Work out the finished part from the listing and answer in its coordinate system (mm). Face numbers are marked on the shaded views. A direction names the side the tool comes from. Give positions to 0.01 mm unless a question says otherwise; leave off trailing zeros. Order: outer loops, then holes, each group sorted by start corner. A loop starts at its lowest first (then second) coordinate and runs counter-clockwise, first axis right, second up.
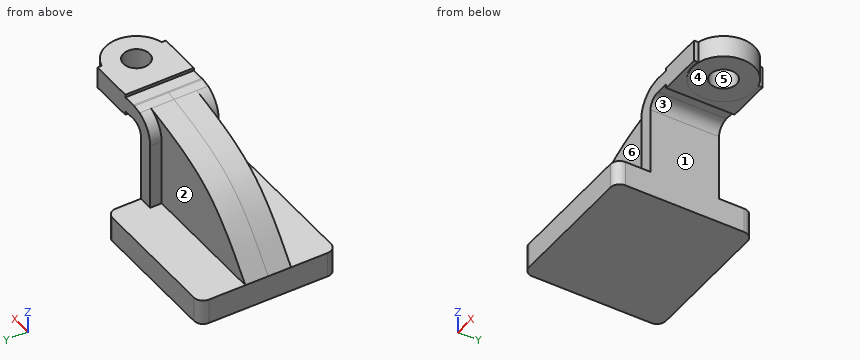
```python
from build123d import *

# Parameters (mm, degrees)
F1_DEPTH = 38.1
F2_DEPTH = 19.05
F3_DEPTH = 12.7
F5_DEPTH = 12.192
F6_R     = 5.08
F7_R     = 7.266587331
F8_DEPTH = 67.1105764264


with BuildPart() as f1:
    # F0 (on Front) → F1 (new body, symmetric)
    with BuildSketch(Plane.XZ):
        Polygon((-40.8368967474, -6.9965338334), (40.8368967474, -6.9965338334), (40.8368967474, 6.9965338334), (32.7088981867, 6.9965338334), (-40.8368967474, 6.9965338334), align=None)
    extrude(amount=F1_DEPTH, both=True)

    # F0 (on Front) → F2 (join, symmetric)
    with BuildSketch(Plane.XZ):
        with BuildLine():
            Line((32.7088981867, 6.9965338334), (40.8368967474, 6.9965338334))
            Line((40.8368967474, 6.9965338334), (40.8368967474, 44.1209748387))
            ThreePointArc((40.8368967474, 44.1209748387), (42.7787364938, 48.6655280984), (47.405064106, 50.403572619))
            Line((47.405064106, 50.403572619), (54.5443966985, 50.403572619))
            Line((54.5443966985, 50.403572619), (54.5443966985, 58.5315711796))
            Line((54.5443966985, 58.5315711796), (47.5487387444, 58.5315711796))
            ThreePointArc((47.5487387444, 58.5315711796), (47.1257024985, 58.5377791506), (46.7026662526, 58.5315711796))
            add(Edge.make_bspline(
                [(42.0115930359, 57.6002229992), (43.5737310544, 57.9125891747), (45.1381986535, 58.2220801772), (46.7026662526, 58.5315711796)],
                knots=[0.9578817781, 0.9578817781, 0.9578817781, 0.9578817781, 1, 1, 1, 1], degree=3))
            ThreePointArc((42.0115930359, 57.6002229992), (35.2603461634, 52.3098432347), (32.7088981867, 44.1209748387))
            Line((32.7088981867, 44.1209748387), (32.7088981867, 6.9965338334))
        make_face()
        Polygon((54.5443966985, 58.5315711796), (54.5443966985, 50.403572619), (54.5443966985, 48.1189936399), (79.1036263108, 48.1189936399), (79.1036263108, 60.113042593), (54.5443966985, 60.113042593), align=None)
    extrude(amount=F2_DEPTH, both=True)

    # F0 (on Front) → F3 (join, symmetric)
    with BuildSketch(Plane.XZ):
        with BuildLine():
            add(Edge.make_bspline(
                [(-40.8368967474, 6.9965338334), (-30.668528225, 20.158177618), (-10.5181051355, 46.2403057616), (24.4122257068, 54.0810415955), (42.0115930359, 57.6002229992)],
                knots=[0, 0, 0, 0, 0.4833692512, 0.9578817781, 0.9578817781, 0.9578817781, 0.9578817781], degree=3))
            Line((-40.8368967474, 6.9965338334), (32.7088981867, 6.9965338334))
            Line((32.7088981867, 6.9965338334), (32.7088981867, 44.1209748387))
            ThreePointArc((32.7088981867, 44.1209748387), (35.2603461634, 52.3098432347), (42.0115930359, 57.6002229992))
        make_face()
    extrude(amount=F3_DEPTH, both=True)

    # F4 (on face) → F5 (join)
    with BuildSketch(Plane.XY.offset(60.113042593)):
        with BuildLine():
            Line((79.1036263108, -16.6910297118), (79.1036263108, 16.6910297118))
            ThreePointArc((79.1036263108, 16.6910297118), (57.6104526514, 0), (79.1036263108, -16.6910297118))
        make_face()
        with BuildLine():
            ThreePointArc((79.1036263108, -16.6910297118), (88.4444418904, -10.5664449916), (92.0654381519, 0))
            ThreePointArc((92.0654381519, 0), (88.4444418904, 10.5664449916), (79.1036263108, 16.6910297118))
            Line((79.1036263108, 16.6910297118), (79.1036263108, -16.6910297118))
        make_face()
    extrude(amount=-F5_DEPTH)

    # F6
    f6_edges = [f1.edges().sort_by_distance(p)[0] for p in [
        (-40.836897, -38.1, 0),
        (40.836897, -38.1, 0),
        (40.836897, 38.1, 0),
        (-40.836897, 38.1, 0),
    ]]
    fillet(f6_edges, radius=F6_R)

    # F7 (on face) → F8 (cut, through all)
    with BuildSketch(Plane.XY.offset(60.113042593)):
        with Locations((74.8379454017, 0)):
            Circle(F7_R)
    extrude(amount=-F8_DEPTH, mode=Mode.SUBTRACT)


solid = f1.part
```
1. The part is cut by section C-C (y = 24). Write down the section's boundary in (x, z), then the cut area to 3 significant figures.
Findings below:
outline: (-40.84, -7) - (40.84, -7) - (40.84, 7) - (-40.84, 7) - close
area: 1,140 mm2
2. Straight lines are drawn through the part: probe 1 along Z at (x, y) = (-2.5, 20); probe 2 along Y at (x, z) = (40, 39.5); probe 3 along Y at (x, z) = (-14, 34.5). For each, find the intervals that lie inside material, in ascending order.
Findings below:
probe 1: z = -7 to 7
probe 2: y = -19.05 to 19.05
probe 3: y = -12.7 to 12.7
3. Given P1, Ø1.9, axis at y = -15.5, z = 28, coming from the -X side; P2, Ø10, axis at x = 43.5, y = 7.5, coming from the +Z side; P3, Ø17, axis at x = 67, y = 3.5, coming from the -Z side; P4, Ø2, axis at x = 58.5, y = -20, coming from the +Z side, each flat-ended and moving along its own axis, determine where each tip first touches the part or whether it passes through.
Findings below:
P1: stops at x = 32.71
P2: stops at z = 58.54
P3: stops at z = 47.92
P4: stops at z = 60.11
4. Which of the six approach directions +Z, -Z, +X, -X, +Y, -Y give full straight-line access (tool end or side, diameter ignored) to the marked faces 1, 2 and 3?
Findings below:
face 1: -Z, +X, +Y, -Y
face 2: +Z, -X, +Y
face 3: -Z, +Y, -Y
5. The part is cut by section A-A (x = 74). Write down the section's boundary in (y, z), then the cut area to 3 significant figures.
Findings below:
outline: (-19.05, 48.12) - (-17.21, 48.12) - (-17.21, 47.92) - (-7.22, 47.92) - (-7.22, 60.11) - (-19.05, 60.11) - close; (7.22, 47.92) - (17.21, 47.92) - (17.21, 48.12) - (19.05, 48.12) - (19.05, 60.11) - (7.22, 60.11) - close
area: 288 mm2
6. The mould has two halves that part along Y. Classify the marked faces 4, 5 and 6: pulls with the +Y half, pulls with the -Y half, needs draft (parallel to the pull), parting line crosses it, or undercut.
Findings below:
face 4: needs draft
face 5: undercut
face 6: pulls with the -Y half
7. The part is cut by section B-B (z = 5). Write down the section's boundary in (x, y).
Findings below:
outline: (-40.84, -33.02) arc R5.08 ccw to (-35.76, -38.1) - (35.76, -38.1) arc R5.08 ccw to (40.84, -33.02) - (40.84, 33.02) arc R5.08 ccw to (35.76, 38.1) - (-35.76, 38.1) arc R5.08 ccw to (-40.84, 33.02) - close
